Source: CAD feature listing. Evaluate the final solid. Frame: model axes, mm. A direction names the side the tool comes from. Round coordinates to 2 decimals unless told otherwise and drop trailing zeros. Order: outer loops, then holes, each group sorted by start corner. A loop starts at its lowest first (then second) coordinate and runs counter-clockwise, first axis right, second up. Notation, with made-up numbers: M 58.25,14 L 87.25,14 A23 ccw 87.25,39 Z; hole C 44,7 d7. An arc over 180 degrees is marked long. Use CSV: the item, a comma, the result in double quotes. Start each with the question number.
```python
from build123d import *

# Parameters (mm, degrees)
SKETCH_1_R      = 18
SKETCH_1_R_2    = 12.5
EXTRUDE_1_DEPTH = 7
SKETCH_3_R      = 18
SKETCH_3_R_2    = 12.5
EXTRUDE_2_DEPTH = 22
EXTRUDE_START   = -14
SKETCH_4_R      = 30
EXTRUDE_3_DEPTH = 7


with BuildPart() as part:
    # Эскиз1 → Вытянуть1 (new body)
    with BuildSketch(Plane.XY):
        Circle(SKETCH_1_R)
        Circle(SKETCH_1_R_2, mode=Mode.SUBTRACT)
    extrude(amount=EXTRUDE_1_DEPTH)

    # Эскиз3 → Вытянуть2 (add)
    with BuildSketch(Plane.XY.offset(7)):
        with Locations(Location((0, 0, 0), (0, 0, 180))):
            Circle(SKETCH_3_R)
        with Locations(Location((0, 0, 0), (0, 0, 180))):
            Circle(SKETCH_3_R_2, mode=Mode.SUBTRACT)
    extrude(amount=EXTRUDE_2_DEPTH)

    # Эскиз4 → Вытянуть3 (add)
    with BuildSketch(Plane(origin=(0, 0, 0), x_dir=(-1, 0, 0), z_dir=(0, 0, -1)).offset(EXTRUDE_START)):
        Circle(SKETCH_4_R)
    extrude(amount=EXTRUDE_3_DEPTH)


solid = part.part
```
(1) Reachability of faces 5 (the face through (-13, -13, 14)), 6 (the face through (0, 0, 7)), 7 (the face through (-12.3, -3.7, 0)) from +Z, -Z, +X, -X, +Y, -Y: full face, straight path, thin tool, end or side. Return the list, or none.
(2) Section D-D on x = 13.5. Return loops of the section in (y, z), plus the area to 3 significant figures.
(3) Line query: line 1 along Y through (x, z) = (0, 24); line 2 along Z through (x, y) = (-3.5, -20); line 3 along Y through (x, z) = (3, 15.5). Output: solid intervals per line, ascending.
(4) Draft query along Y for faces 1 (the face through (-1.627, 12.394, 3.451)), 2 (the face through (13.267, -12.165, 21.395)), 3 (the face through (-11.923, -3.755, 21.395)), 4 (the face through (12.3, 3.7, 29)). Return one class per face: pulls with the +Y half, pulls with the -Y half, needs draft (parallel to the pull), parting line crosses it, or undercut.
(5) Section C-C on z = 26.75. Return loops of the section in (x, y), plus the area to 3 significant figures.
(6) Section A-A on x = 0. Return loops of the section in (y, z).
(7) Contact query for flat-ended pins moving along their axis: P1, Ø4, axis at y = -11, z = 18, coming from the -X side; P2, Ø5, axis at x = 23, z = 3.5, coming from the -Y side; P3, Ø8, axis at y = -7, z = 5.5, coming from the -X side; P4, Ø8, axis at x = -3.5, z = 11, coming from the -Y side. Output: stop coordinate, or through.
Results below:
1,face 5,"+Z"
1,face 6,"-Z"
1,face 7,"-Z, +X, -X, +Y, -Y"
2,outline,"M -26.79,7 L -11.91,7 L -11.91,0 L 11.91,0 L 11.91,7 L 26.79,7 L 26.79,14 L 11.91,14 L 11.91,29 L -11.91,29 L -11.91,14 L -26.79,14 Z"
2,area,"899 mm2"
3,line 1,"y = -18 to -12.5, 12.5 to 18"
3,line 2,"z = 7 to 14"
3,line 3,"y = -17.75 to -12.13, 12.13 to 17.75"
4,face 1,"undercut"
4,face 2,"parting line crosses it"
4,face 3,"undercut"
4,face 4,"needs draft"
5,outline,"C 0,0 d36; hole C 0,0 d25"
5,area,"527 mm2"
6,outline,"M -30,7 L -18,7 L -18,0 L -12.5,0 L -12.5,7 L 12.5,7 L 12.5,0 L 18,0 L 18,7 L 30,7 L 30,14 L 18,14 L 18,29 L 12.5,29 L 12.5,14 L -12.5,14 L -12.5,29 L -18,29 L -18,14 L -30,14 Z"
7,P1,"stops at x = -15.59"
7,P2,"passes through"
7,P3,"stops at x = -29.82"
7,P4,"stops at y = -30"
